Check sheet for the modelled part. Datum: model origin and axes. Units: mm. A direction names the side the tool comes from. Round coordinates to 2 decimals unless told otherwise and drop trailing zeros. Write each loop counter-clockwise with the first axis right and the second up, starting at its lowest first coordinate (ties: lowest second). Pieces come first, ordered by that corner, then holes.
Item 1: Tool access check on faces 1 (the cylindrical face through (4.88, 42.4, 1.08)), 2 (the flat face through (17, 12.66, -18)), 3 (the flat face through (0, 50, 0)). Record the directions out of +Z, -Z, +X, -X, +Y, -Y that give a thin tool (end or side, any length) a straight path to the whole face; none if there is none.
Item 2: Cross-section at B-B on y = 38. Enter the section's corners in (x, z).
Item 3: Cross-section at A-A on y = 17. Enter the section's corners in (x, z), plus the area to 3 significant figures.
Item 4: Material ranges on line 1 (Y direction, x = 14, z = 20.5); line 2 (Y direction, x = -18, z = 15); line 3 (X direction, y = 14, z = 15.5), recorded low to high.
Item 5: Go/stop test with flat-tipped pins: pin 1 Ø6 at (x, z) = (-13, -9) entering from -Y; pin 2 Ø4 at (x, y) = (13, 13) entering from +Z; pin 3 Ø10 at (x, z) = (13, -13.5) entering from -Y. Record where each tip stops, or that it passes through.
from build123d import *

# Parameters (mm, degrees)
FILLET1_R = 50
FILLET2_R = 15


with BuildPart() as part:
    # Sketch2 → Revolve1 (revolve)
    with BuildSketch(Plane(origin=(0, 0, 0), x_dir=(0, 0, -1), z_dir=(1, 0, 0))):
        Polygon((0, 0), (0, 50), (5, 50), (5, 20), (25, 20), (25, 12.660254038), (5, 12.660254038), (5, 8.660254038), align=None)
    revolve(axis=Axis((0, 0, 0), (0, 1, 0)))

    # Fillet1
    # the kernel refuses this fillet: 50 mm, written as the material it adds along each edge
    with BuildSketch(Plane(origin=(0, 12.660254038, 0), x_dir=(0, 0, -1), z_dir=(1, 0, 0))) as fillet1_piece_1:
        with BuildLine():
            CenterArc((24.595917942, -50), FILLET1_R, 90, 23.073918066)
            Line((5, -4), (5, 0))
            Line((5, 0), (24.595917942, 0))
        make_face()
    revolve(axis=Axis((0, 12.660254038, 0), (0, 1, 0)))

    # Fillet2
    fillet2_edges = [part.edges().sort_by_distance(p)[0] for p in [
        (0, 20, 5),
    ]]
    fillet(fillet2_edges, radius=FILLET2_R)


solid = part.part
Response values:
1. face 1: +Y
1. face 2: -Y
1. face 3: +Z, -Z, +X, -X, +Y
2. outline: circle Ø10 at (0, 0)
3. outline: circle Ø50 at (0, 0)
3. area: 1,960 mm2
4. line 1: y = 12.66 to 20
4. line 2: y = 12.65 to 20
4. line 3: x = -19.62 to 19.62
5. pin 1: stops at y = 11.25
5. pin 2: stops at z = 22.45
5. pin 3: stops at y = 11.47
